The listing builds one solid part. Answer for the finished solid, in the listing's coordinates (mm). A direction names the side the tool comes from. Round coordinates to 2 decimals unless told otherwise and drop trailing zeros. Loops run counter-clockwise (first coordinate to the right, second up) from the corner with the lowest first, then second, coordinate; pieces in that order, holes last. Notation, with made-up numbers: (79, 37.5) -> (129, 37.5) arc R34 ccw to (129, 76.5) -> close; hole circle Ø6 at (40, 54). An arc over 180 degrees is marked (long way). Use a Markdown table: item, result. Add a question column.
Q1. Section B-B on x = 50 is taken. Give the vertices of the cut face in (y, z).
Q2. Section C-C on y = -3 is taken. Give the number of separate pieces and of enclosed holes in the cut face, then the cut area to 3 significant figures.
Q3. Section A-A on z = 25 is taken. Give the vertices of the cut face in (x, y), then the cut area to 3 significant figures.
Q4. Consider line 1 (Z direction, x = 65, y = 13.6); line 2 (Z direction, x = 63, y = 3.75); line 3 (Y direction, x = 50, z = -37). Determine where each line is inside the solid, lowest interval first.
Q5. Section D-D on z = -9.5 is taken. Give the vertices of the cut face in (x, y), then the cut area to 3 significant figures.
Q6. For a pull along X with two mould halves and no side action, classify faces 1 (the flat face through (-57, -5, -33.65)), 2 (the cylindrical face through (59.771, -14.514, 36.869)), 3 (the flat face through (37.474, -2.37, 36.741)), 4 (the cylindrical face through (-59.771, -14.514, -36.781)) as released by +X, released by -X, zero draft, split by the parting line, or undercut.
Q7. Given pin 1 Ø3 at (x, y) = (48.5, 2.5) entering from +Z; pin 2 Ø3.5 at (x, z) = (64, 24.5) entering from -Y; pin 3 Ø11 at (x, z) = (-65, 25) entering from -Y; pin 4 Ø8 at (x, z) = (-65, -25) entering from -Y, each flat-ended and moving along its own axis, determine where each tip first touches the part or whether it passes through.
Q8. Which of the six approach directions +Z, -Z, +X, -X, +Y, -Y give full straight-line access (tool end or side, diameter ignored) to faces 5 (the cylindrical face through (34.227, 9.118, 36.047)), 6 (the cylindrical face through (-46.98, -8.81, -36.78)), 7 (the cylindrical face through (51.128, 8.859, 32.447)), 8 (the flat face through (-67, 13, 24))?
from build123d import *

# Parameters (mm, degrees)
CROQUIS1_W                 = 140
CROQUIS1_H                 = 30
SALIENTE_EXTRUIR1_DEPTH    = 40
CORTAR_EXTRUIR1_DEPTH      = 83.006097334
CORTAR_EXTRUIR1_DEPTH_BACK = 83.006097334
CROQUIS2_W                 = 67.3
CROQUIS2_H                 = 25
CROQUIS3_R                 = 6.55
CORTAR_EXTRUIR2_DEPTH      = 80
CORTAR_EXTRUIR3_REACH      = 86.41
CROQUIS4_R                 = 1.651
CROQUIS5_R                 = 3.5
CROQUIS5_R_2               = 1.651
CORTAR_EXTRUIR4_DEPTH      = 3
CORTAR_EXTRUIR5_DEPTH      = 83.006097334
CORTAR_EXTRUIR5_DEPTH_BACK = 83.006097334
REDONDEO1_R                = 4


with BuildPart() as part:
    # Croquis1 → Saliente-Extruir1 (new, symmetric)
    with BuildSketch(Plane.XY):
        Rectangle(CROQUIS1_W, CROQUIS1_H)
    extrude(amount=SALIENTE_EXTRUIR1_DEPTH, both=True)

    # Croquis2 → Cortar-Extruir1 (cut, two sides: drawn at the far end of the back side and taken through both)
    with BuildSketch(Plane(origin=(0, 0, 0), x_dir=(0, 0, -1), z_dir=(1, 0, 0)).offset(-CORTAR_EXTRUIR1_DEPTH_BACK)):
        with Locations((0, -2.5)):
            Rectangle(CROQUIS2_W, CROQUIS2_H)
    extrude(amount=CORTAR_EXTRUIR1_DEPTH + CORTAR_EXTRUIR1_DEPTH_BACK, mode=Mode.SUBTRACT)

    # Croquis3 → Cortar-Extruir2 (cut)
    with BuildSketch(Plane.XY.offset(40)):
        with Locations((50, -3)):
            Circle(CROQUIS3_R)
        with Locations((-50, -3)):
            Circle(CROQUIS3_R)
    extrude(amount=-CORTAR_EXTRUIR2_DEPTH, mode=Mode.SUBTRACT)

    # Croquis4 → Cortar-Extruir3 (cut, up to next)
    with BuildSketch(Plane.XZ.offset(-10), mode=Mode.PRIVATE) as cortar_extruir3_sk1:
        with Locations(Location((-65, 25, 0), (0, 0, 270))):
            Circle(CROQUIS4_R)
    cortar_extruir3_tool1 = extrude(cortar_extruir3_sk1.sketch, amount=-CORTAR_EXTRUIR3_REACH, mode=Mode.PRIVATE) & part.part
    # Croquis4 → Cortar-Extruir3 (cut, up to next)
    with BuildSketch(Plane.XZ.offset(-10), mode=Mode.PRIVATE) as cortar_extruir3_sk2:
        with Locations(Location((-65, -25, 0), (0, 0, 270))):
            Circle(CROQUIS4_R)
    cortar_extruir3_tool2 = extrude(cortar_extruir3_sk2.sketch, amount=-CORTAR_EXTRUIR3_REACH, mode=Mode.PRIVATE) & part.part
    cortar_extruir3_1 = cortar_extruir3_tool1.solids().sort_by_distance((-65, 10, 25))[0]
    add(cortar_extruir3_1, mode=Mode.SUBTRACT)
    cortar_extruir3_2 = cortar_extruir3_tool2.solids().sort_by_distance((-65, 10, -25))[0]
    add(cortar_extruir3_2, mode=Mode.SUBTRACT)
    cortar_extruir3 = cortar_extruir3_1 + cortar_extruir3_2  # Cortar-Extruir3 as one shape, for the pattern or mirror that repeats it

    # Croquis5 → Cortar-Extruir4 (cut)
    # profile 1 of 2: a face of its own
    with BuildSketch(Plane.XZ.offset(-10)):
        with Locations(Location((-65, 25, 0), (0, 0, 270))):
            Circle(CROQUIS5_R)
        with Locations(Location((-65, 25, 0), (0, 0, 270))):
            Circle(CROQUIS5_R_2, mode=Mode.SUBTRACT)
    # profile 2 of 2: a face of its own
    with BuildSketch(Plane.XZ.offset(-10)):
        with Locations(Location((-65, -25, 0), (0, 0, 270))):
            Circle(CROQUIS5_R)
        with Locations(Location((-65, -25, 0), (0, 0, 270))):
            Circle(CROQUIS5_R_2, mode=Mode.SUBTRACT)
    cortar_extruir4 = extrude(amount=-CORTAR_EXTRUIR4_DEPTH, mode=Mode.SUBTRACT)

    # Croquis9 → Cortar-Extruir5 (cut, two sides: drawn at the far end of the back side and taken through both)
    with BuildSketch(Plane.XY.offset(-CORTAR_EXTRUIR5_DEPTH_BACK)):
        Polygon((-40, -15), (-35, 10), (35, 10), (40, -15), align=None)
        Polygon((-70, 0), (-60, -15), (-70, -15), align=None)
        Polygon((70, 0), (60, -15), (70, -15), align=None)
    extrude(amount=CORTAR_EXTRUIR5_DEPTH + CORTAR_EXTRUIR5_DEPTH_BACK, mode=Mode.SUBTRACT)

    # Simetría4: Cortar-Extruir3, Cortar-Extruir4 across plane
    add(cortar_extruir3.mirror(Plane(origin=(0, 0, 0), x_dir=(0, 0, 1), z_dir=(1, 0, 0))), mode=Mode.SUBTRACT)
    add(cortar_extruir4.mirror(Plane(origin=(0, 0, 0), x_dir=(0, 0, 1), z_dir=(1, 0, 0))), mode=Mode.SUBTRACT)

    # Redondeo1
    redondeo1_edges = [part.edges().sort_by_distance(p)[0] for p in [
        (-70, 0, 36.825),
        (-70, 0, -36.825),
        (-60, -15, 36.825),
        (-60, -15, -36.825),
        (70, 0, 36.825),
        (70, 0, -36.825),
        (60, -15, 36.825),
        (60, -15, -36.825),
        (-52.5, 10, 33.65),
        (-52.5, 10, -33.65),
        (52.5, 10, -33.65),
        (52.5, 10, 33.65),
        (40, -15, 36.825),
        (40, -15, -36.825),
        (-40, -15, 36.825),
        (-40, -15, -36.825),
        (-35, 10, 36.825),
        (-35, 10, -36.825),
        (35, 10, 36.825),
        (35, 10, -36.825),
    ]]
    fillet(redondeo1_edges, radius=REDONDEO1_R)


solid = part.part
Checked values:
| question | item | result |
|---|---|---|
| 1 | outline | (-15, -40) -> (-9.55, -40) -> (-9.55, -33.65) -> (-15, -33.65) -> close; (-15, 33.65) -> (-9.55, 33.65) -> (-9.55, 40) -> (-15, 40) -> close; (3.55, -40) -> (15, -40) -> (15, 40) -> (3.55, 40) -> (3.55, 33.65) -> (6, 33.65) arc R4 cw to (10, 29.65) -> (10, -29.65) arc R4 cw to (6, -33.65) -> (3.55, -33.65) -> close |
| 2 | separate pieces | 8 |
| 2 | enclosed holes | 0 |
| 2 | area | 439 mm2 |
| 3 | outline | (-70, 10) -> (-68.5, 10) -> (-68.5, 13) -> (-66.65, 13) -> (-66.65, 15) -> (-70, 15) -> close; (-63.35, 13) -> (-61.5, 13) -> (-61.5, 10) -> (61.5, 10) -> (61.5, 13) -> (63.35, 13) -> (63.35, 15) -> (-63.35, 15) -> close; (66.65, 13) -> (68.5, 13) -> (68.5, 10) -> (70, 10) -> (70, 15) -> (66.65, 15) -> close |
| 3 | area | 645 mm2 |
| 4 | line 1 | z = -40 to -26.65, -23.35 to 23.35, 26.65 to 40 |
| 4 | line 2 | z = -40 to -33.65, 33.65 to 40 |
| 4 | line 3 | y = -15 to -9.55, 3.55 to 15 |
| 5 | outline | (-70, 10) -> (70, 10) -> (70, 15) -> (-70, 15) -> close |
| 5 | area | 700 mm2 |
| 6 | face 1 | zero draft |
| 6 | face 2 | released by +X |
| 6 | face 3 | undercut |
| 6 | face 4 | released by -X |
| 7 | pin 1 | stops at z = 40 |
| 7 | pin 2 | stops at y = 13 |
| 7 | pin 3 | stops at y = 9.91 |
| 7 | pin 4 | stops at y = 10 |
| 8 | face 5 | +Z, -Z, -Y |
| 8 | face 6 | +Z, -Z |
| 8 | face 7 | +X, -X, -Y |
| 8 | face 8 | -Y |
